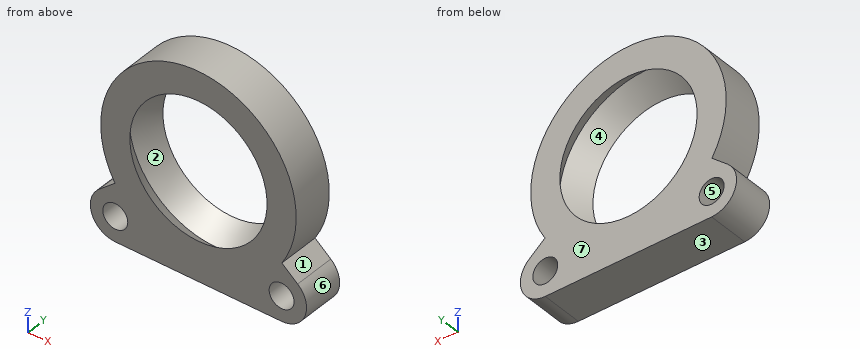
from build123d import *

# Parameters (mm, degrees)
SKETCH017_R  = 1.5
PAD008_DEPTH = 2.5


with BuildPart() as outerbearing:
    # Sketch007 → Revolution001 (revolve)
    with BuildSketch(Plane.YZ):
        Polygon((-2.5, 8.251111), (0, 10.34886), (2.5, 8.251111), (2.5, 11.751111), (-2.5, 11.751111), align=None)
    revolve(axis=Axis((0, 0, 0), (0, 1, 0)))


with BuildPart() as fusion001:
    # Sketch017 → Pad008 (new body, symmetric)
    with BuildSketch(Plane.XZ):
        with BuildLine():
            ThreePointArc((-9.84093, -5.950302), (0, -11.5), (9.84093, -5.950302))
            Line((11.928352, -7.701857), (9.84093, -5.950302))
            ThreePointArc((9.999998, -13), (12.81908, -11.026055), (11.928352, -7.701857))
            Line((-10, -13), (9.999998, -13))
            ThreePointArc((-11.928369, -7.701871), (-12.819077, -11.026064), (-10, -13))
            Line((-9.84093, -5.950302), (-11.928369, -7.701871))
        make_face()
        with Locations((10, -10)):
            Circle(SKETCH017_R, mode=Mode.SUBTRACT)
        with Locations((-10, -10)):
            Circle(SKETCH017_R, mode=Mode.SUBTRACT)
    extrude(amount=PAD008_DEPTH, both=True)

    # Fusion001: union OuterBearing
    add(outerbearing.part)


solid = fusion001.part
Design review of the part built by this model. Coordinates are the model's own, in mm. Face numbers are marked on the shaded views. A direction names the side the tool comes from. Round coordinates to 2 decimals unless told otherwise and drop trailing zeros. Write each loop counter-clockwise with the first axis right and the second up, starting at its lowest first coordinate (ties: lowest second). Pieces come first, ordered by that corner, then holes. Notation, with made-up numbers: (60, 81.5) -> (99, 81.5) arc R22 cw to (99, 94.5) -> close; hole circle Ø1 at (6.25, 37.5). An arc over 180 degrees is marked (long way). One line per item, written item: value. Start each with the question number.
Q1. To check wall thickness, follow probe 1 along X at (y, z) = (-1.8, -9.75); probe 2 along X at (y, z) = (-1.6, -5); probe 3 along Y at (x, z) = (-6, 6). State the ranges of each line that lie inside material, in increasing order.
Q2. Tool access review of the marked faces 1, 2 and 3: name each direction out of +Z, -Z, +X, -X, +Y, -Y from which nothing blocks a thin tool from reaching the whole face with its end or side.
Q3. Add section C-C (z = 0). Give the boundary of the cut face in (x, y), then the cut area to 3 significant figures.
Q4. Insertion check: P1, Ø1.5, axis at y = 1.5, z = -8, coming from the -X side; P2, Ø1, axis at y = 1, z = 9, coming from the -X side; P3, Ø3, axis at x = 2, y = 1, coming from the +Z side. Each pin has a flat end and moves straight along its axis. Give the tip position at first contact, or say it passes through.
Q5. Add section D-D (x = -11). Give the boundary of the cut face in (y, z), then the cut area to 3 significant figures.
Q6. The part is to be moulded in two halves that separate along X. For the marked faces 4, 5, 6 and 7, say which applies: pulls with the +X half, pulls with the -X half, needs draft (parallel to the pull), parting line crosses it, or undercut.
Q7. Add section B-B (y = -0.55). Give the boundary of the cut face in (x, z).
Q8. Add section A-A (x = 0). Give the boundary of the cut face in (y, z).
Response:
1. probe 1: x = -12.99 to -11.48, -8.52 to 8.52, 11.48 to 12.99
1. probe 2: x = -10.63 to -7.49, 7.49 to 10.63
1. probe 3: y = -2.5 to -2.22, 2.22 to 2.5
2. face 1: +X, +Y, -Y
2. face 2: none
2. face 3: -Z, +X, -X, +Y, -Y
3. outline: (-11.75, -2.5) -> (-8.25, -2.5) -> (-10.35, 0) -> (-8.25, 2.5) -> (-11.75, 2.5) -> close; (8.25, -2.5) -> (11.75, -2.5) -> (11.75, 2.5) -> (8.25, 2.5) -> (10.35, 0) -> close
3. area: 24.5 mm^2
4. P1: stops at x = -12.73
4. P2: stops at x = -8.11
4. P3: stops at z = 11.74
5. outline: (-2.5, -12.83) -> (2.5, -12.83) -> (2.5, -11.12) -> (-2.5, -11.12) -> close; (-2.5, -8.88) -> (2.5, -8.88) -> (2.5, -6.92) -> (-2.5, -6.92) -> close; (-2.5, -4.13) -> (2.5, -4.13) -> (2.5, 4.13) -> (-2.5, 4.13) -> close
5. area: 59.7 mm^2
6. face 4: undercut
6. face 5: undercut
6. face 6: pulls with the +X half
6. face 7: needs draft
7. outline: (-11.93, -7.7) arc R3 ccw to (-10, -13) -> (10, -13) arc R3 ccw to (11.93, -7.7) -> (10.04, -6.11) arc R11.75 ccw (long way) to (-10.04, -6.11) -> close; hole circle Ø3 at (-10, -10); hole circle Ø19.77 at (0, 0); hole circle Ø3 at (10, -10)
8. outline: (-2.5, -13) -> (2.5, -13) -> (2.5, -8.25) -> (0, -10.35) -> (-2.5, -8.25) -> close; (-2.5, 8.25) -> (0, 10.35) -> (2.5, 8.25) -> (2.5, 11.75) -> (-2.5, 11.75) -> close
